```python
from build123d import *

# Parameters (mm, degrees)
BOSS_EXTRUDE1_DEPTH     = 3.175
CUT_EXTRUDE1_DEPTH      = 120.85362166
CUT_EXTRUDE1_DEPTH_BACK = 120.85362166
CUT_EXTRUDE2_DEPTH      = 213.914467862
CUT_EXTRUDE2_DEPTH_BACK = 213.914467862


with BuildPart() as part:
    # Sketch1 → Boss-Extrude1 (new body)
    with BuildSketch(Plane.YZ):
        Polygon((0, 0), (203.2, 0), (203.2, 63.5), (101.6, 63.5), align=None)
    extrude(amount=BOSS_EXTRUDE1_DEPTH)

    # Sketch2 → Cut-Extrude1 (cut, two sides: drawn at the far end of the back side and taken through both)
    with BuildSketch(Plane(origin=(0, 101.6, 63.5), x_dir=(-1, 0, 0), z_dir=(0, 0.8479983040050879, 0.52999894000318)).offset(-CUT_EXTRUDE1_DEPTH_BACK)):
        Polygon((-3.175, -8.683746968), (-3.175, 1.50596977), (0, 1.50596977), (0, -8.683746968), (-1.5875, 0), align=None)
    extrude(amount=CUT_EXTRUDE1_DEPTH + CUT_EXTRUDE1_DEPTH_BACK, mode=Mode.SUBTRACT)

    # Sketch3 → Cut-Extrude2 (cut, two sides: drawn at the far end of the back side and taken through both)
    with BuildSketch(Plane.XY.offset(63.5).offset(-CUT_EXTRUDE2_DEPTH_BACK)):
        Polygon((0, 198.707072367), (1.5875, 203.2), (3.175, 198.707072367), (3.175, 209.769975366), (0, 209.769975366), align=None)
    extrude(amount=CUT_EXTRUDE2_DEPTH + CUT_EXTRUDE2_DEPTH_BACK, mode=Mode.SUBTRACT)


solid = part.part
```
Check sheet for the modelled part. Datum: model origin and axes. Units: mm. Round coordinates to 2 decimals unless told otherwise and drop trailing zeros. Order: outer loops, then holes, each group sorted by start corner. A loop starts at its lowest first (then second) coordinate and runs counter-clockwise, first axis right, second up. Notation, with made-up numbers: (12, 26) -> (21, 26) arc R10 ccw to (21, 36) -> close; hole circle Ø10 at (13.5, 32). An arc over 180 degrees is marked (long way). One line per item, written item: value. Start each with the question number.
Q1. Cross-section at B-B (z = 57). Record the boundary of the cut face in (x, y) (1 decimal), and give its area (3 significant figures).
Q2. Cross-section at C-C (x = 2.65). Record the boundary of the cut face in (y, z), and give its area (3 significant figures).
Q3. Gauge pin test, flat ends, axial feed: pin 1 Ø8 at (y, z) = (73, 43.5) entering from +X; pin 2 Ø1 at (y, z) = (63.5, 40) entering from +X; pin 3 Ø2 at (y, z) = (58, 34.5) entering from -X. Record the tip position at first contact, or that the pin passes through.
Q4. Cross-section at A-A (y = 55). Record the boundary of the cut face in (x, z) (1 decimal).
Q5. Mould release check, pull along Y, two halves, no side actions. Record for faces 1 (the face through (0, 127, 25)), 2 (the face through (0.783, 58.231, 31.202)), 3 (the face through (0.78, 200.92, 31.31)): pulls with the +Y half, pulls with the -Y half, needs draft (parallel to the pull), parting line crosses it, or undercut.
Q6. Cross-section at D-D (y = 85). Record the boundary of the cut face in (x, z) (1 decimal), and give its area (3 significant figures).
Completed:
1. outline: (0, 107.6) -> (1.6, 91.2) -> (3.2, 107.6) -> (3.2, 198.7) -> (1.6, 203.2) -> (0, 198.7) -> close
1. area: 322 mm²
2. outline: (10.97, 0) -> (200.19, 0) -> (200.19, 63.5) -> (112.57, 63.5) -> close
2. area: 8,790 mm²
3. pin 1: stops at x = 2.65
3. pin 2: stops at x = 1.63
3. pin 3: stops at x = 1.13
4. outline: (0, 0) -> (3.2, 0) -> (3.2, 24.1) -> (1.6, 34.4) -> (0, 24.1) -> close
5. face 1: needs draft
5. face 2: pulls with the -Y half
5. face 3: pulls with the +Y half
6. outline: (0, 0) -> (3.2, 0) -> (3.2, 42.9) -> (1.6, 53.1) -> (0, 42.9) -> close
6. area: 152 mm²
